Input: part model. Units: mm. Frame: model coordinates. A direction names the side the tool comes from. Coordinates: 2 decimals unless noted, no trailing zeros. Loops run counter-clockwise (first coordinate to the right, second up) from the corner with the lowest first, then second, coordinate; pieces in that order, holes last. Notation, with made-up numbers: (49, -8) -> (55, -8) arc R14 cw to (55, 17) -> close; hole circle Ø5 at (11, -38). An arc over 180 degrees is marked (long way). Put each result on its own line as item: value. Start each with the question number.
1) Contact query for flat-ended pins moving along their axis: P1, Ø2.5, axis at y = 77, z = 1.5, coming from the +X side; P2, Ø1.5, axis at x = -80, z = 1.5, coming from the -Y side; P3, Ø1, axis at x = -101, z = 4.5, coming from the +Y side. Output: stop coordinate, or through.
2) Cut plane A-A (z = 1.25). Return the cut outline in (x, y), plus the area to 3 significant figures.
3) Cut plane B-B (x = -116.5). Return the cut outline in (y, z), plus the area to 3 significant figures.
4) Set-up query: faces 1 (the flat face through (-99.858, 155, 3)), 2 (the flat face through (-123, 79.059, 2)), 3 (the flat face through (-84.858, 77, 3)), 4 (the flat face through (-167, 152.059, 2)), 5 (the flat face through (-77, 152.059, 2)). Return all of +Z, -Z, +X, -X, +Y, -Y with unobstructed straight access to the full face (end or side cutting, diameter ignored); none if empty.
5) Pull-direction query (X, two-part tool) for faces 6 (the flat face through (-69.858, 115, 2)), 7 (the flat face through (-159.858, 155, 3)), 8 (the cylindrical face through (-168.473, 86.485, 2.535)); classes: pulls with the +X half, pulls with the -X half, needs draft (parallel to the pull), parting line crosses it, or undercut.
6) Material intervals for L1, parallel to Y at x = -169, z = 4.5; L2, parallel to Y at x = -102.5, z = 2.05; L3, parallel to Y at x = -79, z = 2.25, sorted ascending.
from build123d import *

# Parameters (mm, degrees)
ESQUISSE1_W             = 105
ESQUISSE1_H             = 73
BOSS_EXTRU_1_DEPTH      = 5
ESQUISSE2_R             = 1.5
ENL_V_MAT_EXTRU_1_DEPTH = 5
ESQUISSE3_W             = 15
ESQUISSE3_H             = 5
BOSS_EXTRU_2_DEPTH      = 5


with BuildPart() as part:
    # Esquisse1 → Boss.-Extru.1 (new body)
    with BuildSketch(Plane.XY):
        with Locations((-122.358209677, 115.559145013)):
            Rectangle(ESQUISSE1_W, ESQUISSE1_H)
    extrude(amount=BOSS_EXTRU_1_DEPTH)

    # Esquisse2 → Enlèv. mat.-Extru.1 (cut)
    with BuildSketch(Plane.XY.offset(5)):
        with Locations((-101.358209677, 122.559145013)):
            Circle(ESQUISSE2_R)
        with Locations((-169.858209677, 122.559145013)):
            Circle(ESQUISSE2_R)
        with Locations((-169.858209677, 87.059145013)):
            Circle(ESQUISSE2_R)
        with Locations((-101.358209677, 87.059145013)):
            Circle(ESQUISSE2_R)
    extrude(amount=-ENL_V_MAT_EXTRU_1_DEPTH, mode=Mode.SUBTRACT)

    # Esquisse3 → Boss.-Extru.2 (add)
    with BuildSketch(Plane.XY.offset(5)):
        with Locations((-152.358209677, 76.559145013)):
            Rectangle(ESQUISSE3_W, ESQUISSE3_H)
        with Locations((-92.358209677, 76.559145013)):
            Rectangle(ESQUISSE3_W, ESQUISSE3_H)
        with Locations((-92.358209677, 154.559145013)):
            Rectangle(ESQUISSE3_W, ESQUISSE3_H)
        with Locations((-152.358209677, 154.559145013)):
            Rectangle(ESQUISSE3_W, ESQUISSE3_H)
    extrude(amount=-BOSS_EXTRU_2_DEPTH)


solid = part.part
Results found:
1. P1: stops at x = -84.86
1. P2: stops at y = 79.06
1. P3: stops at y = 152.06
2. outline: (-174.86, 79.06) -> (-159.86, 79.06) -> (-159.86, 74.06) -> (-144.86, 74.06) -> (-144.86, 79.06) -> (-99.86, 79.06) -> (-99.86, 74.06) -> (-84.86, 74.06) -> (-84.86, 79.06) -> (-69.86, 79.06) -> (-69.86, 152.06) -> (-84.86, 152.06) -> (-84.86, 157.06) -> (-99.86, 157.06) -> (-99.86, 152.06) -> (-144.86, 152.06) -> (-144.86, 157.06) -> (-159.86, 157.06) -> (-159.86, 152.06) -> (-174.86, 152.06) -> close; hole circle Ø3 at (-169.86, 87.06); hole circle Ø3 at (-169.86, 122.56); hole circle Ø3 at (-101.36, 87.06); hole circle Ø3 at (-101.36, 122.56)
2. area: 7,940 mm2
3. outline: (79.06, 0) -> (152.06, 0) -> (152.06, 5) -> (79.06, 5) -> close
3. area: 365 mm2
4. face 1: +Z, -Z, +Y
4. face 2: +Z, -Z, -Y
4. face 3: +Z, -Z, +X, -Y
4. face 4: +Z, -Z, -X, +Y
4. face 5: +Z, -Z, +X, +Y
5. face 6: pulls with the +X half
5. face 7: pulls with the -X half
5. face 8: undercut
6. L1: y = 79.06 to 85.83, 88.29 to 121.33, 123.79 to 152.06
6. L2: y = 79.06 to 86.09, 88.03 to 121.59, 123.53 to 152.06
6. L3: y = 79.06 to 152.06
